```python
from build123d import *

# Parameters (mm, degrees)
F0_R     = 76.2
F0_R_2   = 4.826
F1_DEPTH = 3.175
F3_DEPTH = 25.4


with BuildPart() as f1:
    # F0 (on Front) → F1 (new body)
    with BuildSketch(Plane.XZ):
        Circle(F0_R)
        with BuildLine():
            ThreePointArc((-57.15, -6.35), (-40.659839, -40.659839), (-6.35, -57.15))
            Line((-6.35, -57.15), (-6.35, -69.85))
            ThreePointArc((-6.35, -69.85), (-49.595085, -49.595085), (-69.85, -6.35))
            Line((-69.85, -6.35), (-57.15, -6.35))
        make_face(mode=Mode.SUBTRACT)
        with BuildLine():
            Line((-31.75, -6.35), (-17.526, -6.35))
            ThreePointArc((-17.526, -6.35), (-13.181107, -13.181107), (-6.35, -17.526))
            Line((-6.35, -17.526), (-6.35, -31.75))
            ThreePointArc((-6.35, -31.75), (-22.895251, -22.895251), (-31.75, -6.35))
        make_face(mode=Mode.SUBTRACT)
        with BuildLine():
            Line((6.35, -31.75), (6.35, -17.526))
            ThreePointArc((6.35, -17.526), (13.181107, -13.181107), (17.526, -6.35))
            Line((17.526, -6.35), (31.75, -6.35))
            ThreePointArc((31.75, -6.35), (22.895251, -22.895251), (6.35, -31.75))
        make_face(mode=Mode.SUBTRACT)
        with BuildLine():
            ThreePointArc((6.35, -57.15), (40.659839, -40.659839), (57.15, -6.35))
            Line((57.15, -6.35), (69.85, -6.35))
            ThreePointArc((69.85, -6.35), (49.595085, -49.595085), (6.35, -69.85))
            Line((6.35, -69.85), (6.35, -57.15))
        make_face(mode=Mode.SUBTRACT)
        with BuildLine():
            Line((-6.35, 31.75), (-6.35, 17.526))
            ThreePointArc((-6.35, 17.526), (-13.181107, 13.181107), (-17.526, 6.35))
            Line((-17.526, 6.35), (-31.75, 6.35))
            ThreePointArc((-31.75, 6.35), (-22.895251, 22.895251), (-6.35, 31.75))
        make_face(mode=Mode.SUBTRACT)
        with BuildLine():
            ThreePointArc((-6.35, 57.15), (-40.659839, 40.659839), (-57.15, 6.35))
            Line((-57.15, 6.35), (-69.85, 6.35))
            ThreePointArc((-69.85, 6.35), (-49.595085, 49.595085), (-6.35, 69.85))
            Line((-6.35, 69.85), (-6.35, 57.15))
        make_face(mode=Mode.SUBTRACT)
        Circle(F0_R_2, mode=Mode.SUBTRACT)
        with BuildLine():
            Line((31.75, 6.35), (17.526, 6.35))
            ThreePointArc((17.526, 6.35), (13.181107, 13.181107), (6.35, 17.526))
            Line((6.35, 17.526), (6.35, 31.75))
            ThreePointArc((6.35, 31.75), (22.895251, 22.895251), (31.75, 6.35))
        make_face(mode=Mode.SUBTRACT)
        with BuildLine():
            ThreePointArc((57.15, 6.35), (40.659839, 40.659839), (6.35, 57.15))
            Line((6.35, 57.15), (6.35, 69.85))
            ThreePointArc((6.35, 69.85), (49.595085, 49.595085), (69.85, 6.35))
            Line((69.85, 6.35), (57.15, 6.35))
        make_face(mode=Mode.SUBTRACT)
    extrude(amount=F1_DEPTH)

    # F2 (on face) → F3 (cut)
    with BuildSketch(Plane.XZ.offset(3.175)):
        Polygon((-81.831723, 12.460574), (-65.217622, 12.460574), (-44.52287, 45.105822), (-14.500901, 64.343199), (-12.169099, 78.916967), (-54.433033, 65.509103), align=None)
        Polygon((12.314837, 79.499915), (12.314837, 63.468769), (44.668611, 47.146149), (63.323036, 15.083852), (85.183688, 15.083852), (62.157135, 64.634673), align=None)
        Polygon((91.596149, -12.02336), (63.61451, -12.02336), (48.457786, -43.794177), (12.314837, -60.991228), (12.314837, -79.354182), (57.15, -66.820741), align=None)
        Polygon((-12.169099, -78.771226), (-12.169099, -63.5), (-48.312049, -43.794177), (-63.177295, -12.02336), (-81.248775, -12.02336), (-76.87664, -30.969264), (-63.177295, -60.991228), align=None)
    extrude(amount=-F3_DEPTH, mode=Mode.SUBTRACT)


solid = f1.part
```
Geometry: final body of the model. Coordinates: model frame, mm. A direction names the side the tool comes from. Round coordinates to 2 decimals unless told otherwise and drop trailing zeros. Loops run counter-clockwise (first coordinate to the right, second up) from the corner with the lowest first, then second, coordinate; pieces in that order, holes last. Notation, with made-up numbers: (-13.75, 25) -> (14.25, 25) arc R26 ccw to (14.25, 64) -> close; hole circle Ø7 at (28.5, -39). An arc over 180 degrees is marked (long way). Write each question's results on one line, items separated by ' | '.
Item 1: Set-up query: faces 3 (the face through (-1, -3.175, 18)), 4 (the face through (-13.1, -1.57, 13.26)). Return all of +Z, -Z, +X, -X, +Y, -Y with unobstructed straight access to the full face (end or side cutting, diameter ignored); none if empty.
Answers below:
face 3: +Z, -Z, +X, -X, -Y | face 4: +Y, -Y
Item 2: Line query: probe 1 along X at (y, z) = (-2.45, -29); probe 2 along Z at (x, y) = (0, -1.65); probe 3 along X at (y, z) = (-0.2, -8.5). Output: solid intervals per line, ascending. Write a range as [from, to].
Answers below:
probe 1: x = [-49.65, -14.4], [-6.35, 6.35], [14.4, 49.65] | probe 2: z = [-76.2, -4.83], [4.83, 76.2] | probe 3: x = [-75.72, -69.62], [-56.87, -31.24], [-16.59, 16.59], [31.24, 56.87], [69.62, 75.72]
Item 3: Cut plane D-D on z = -22. Return the cut outline in (x, y) (3 decimals).
Answers below:
outline: (-53.127, -3.175) -> (-23.757, -3.175) -> (-23.757, 0) -> (-53.127, 0) -> close; (-6.35, -3.175) -> (6.35, -3.175) -> (6.35, 0) -> (-6.35, 0) -> close; (23.757, -3.175) -> (53.127, -3.175) -> (53.127, 0) -> (23.757, 0) -> close
Item 4: Cut plane A-A on z = 0. Return the cut outline in (x, y) (3 decimals).
Answers below:
outline: (-76.2, -3.175) -> (-4.826, -3.175) -> (-4.826, 0) -> (-76.2, 0) -> close; (4.826, -3.175) -> (76.2, -3.175) -> (76.2, 0) -> (4.826, 0) -> close
Item 5: Cut plane C-C on x = 20. Return the cut outline in (y, z) (3 decimals).
Answers below:
outline: (-3.175, -53.911) -> (0, -53.911) -> (0, -25.463) -> (-3.175, -25.463) -> close; (-3.175, -6.35) -> (0, -6.35) -> (0, 6.35) -> (-3.175, 6.35) -> close; (-3.175, 25.463) -> (0, 25.463) -> (0, 53.911) -> (-3.175, 53.911) -> close
Item 6: Cut plane B-B on x = 0. Return the cut outline in (y, z) (3 decimals).
Answers below:
outline: (-3.175, -76.2) -> (0, -76.2) -> (0, -4.826) -> (-3.175, -4.826) -> close; (-3.175, 4.826) -> (0, 4.826) -> (0, 76.2) -> (-3.175, 76.2) -> close
Item 7: Pull-direction query (Z, two-part tool) for faces 1 (the face through (-1, 0, 18)), 2 (the face through (13.26, -1.57, 13.1)); classes: pulls with the +Z half, pulls with the -Z half, needs draft (parallel to the pull), parting line crosses it, or undercut.
Answers below:
face 1: needs draft | face 2: undercut
Item 8: Pin query (flat end, axial travel): pin 1 Ø1.6 at (x, y) = (63.5, -1.5) entering from +Z; pin 2 Ø1 at (x, y) = (65, -1.5) entering from -Z; pin 3 Ø1 at (x, y) = (22, -1) entering from +Z. Return the tip coordinate at first contact, or that it passes through.
Answers below:
pin 1: stops at z = 6.35 | pin 2: stops at z = -6.35 | pin 3: stops at z = 53.33
